```python
from build123d import *

# Parameters (mm, degrees)
CROQUIS1_R                                           = 8.5
SALIENTE_EXTRUIR1_DEPTH                              = 6
SALIENTE_EXTRUIR2_DEPTH                              = 5
REFRENTADO_PARA_TORNILLO_CON_CABEZA_TRON_D           = 4.5
REFRENTADO_PARA_TORNILLO_CON_CABEZA_TRON_CBORE_D     = 6
REFRENTADO_PARA_TORNILLO_CON_CABEZA_TRON_CBORE_DEPTH = 3.1
CHAFL_N1_SIZE                                        = 5
REDONDEO1_R                                          = 10
CHAFL_N2_SIZE                                        = 2
REDONDEO2_R                                          = 5
REDONDEO3_R                                          = 5
REDONDEO4_R                                          = 5
REDONDEO5_R                                          = 5


with BuildPart() as part:
    # Croquis1 → Saliente-Extruir1 (new body)
    with BuildSketch(Plane.XY):
        Polygon((-22.5, 0), (22.5, 0), (22.5, 17), (13, 17), (13, 34), (-13, 34), (-13, 17), (-22.5, 17), align=None)
        with Locations((0, 22)):
            Circle(CROQUIS1_R, mode=Mode.SUBTRACT)
    extrude(amount=SALIENTE_EXTRUIR1_DEPTH)

    # Croquis2 → Saliente-Extruir2 (add)
    with BuildSketch(Plane.XY.offset(6)):
        Polygon((22.5, 0), (22.5, 17), (13, 17), (13, 34), (-13, 34), (-13, 17), (-22.5, 17), (-22.5, 0), align=None)
    extrude(amount=SALIENTE_EXTRUIR2_DEPTH)

    # Refrentado para tornillo con cabeza troncocónica de M41 (through all)
    with Locations(Plane(origin=(17, 17, 5.5), x_dir=(1, 0, 0), z_dir=(0, 1, 0))):
        with Locations((0, 0), (-34, 0)):
            CounterBoreHole(REFRENTADO_PARA_TORNILLO_CON_CABEZA_TRON_D / 2, REFRENTADO_PARA_TORNILLO_CON_CABEZA_TRON_CBORE_D / 2, REFRENTADO_PARA_TORNILLO_CON_CABEZA_TRON_CBORE_DEPTH)

    # Chaflán1
    # the kernel refuses this chamfer: 5 mm, written as the material it adds along each edge
    with BuildSketch(Plane(origin=(-13, 17, 11), x_dir=(-0.9996219169112968, -0.02749587661058561, 0), z_dir=(0, 0, -1))) as chafl_n1_piece_1_section:
        Polygon((CHAFL_N1_SIZE * 0.999621916911, CHAFL_N1_SIZE * 0.0274958766106), (-CHAFL_N1_SIZE * 0.0274958766106, CHAFL_N1_SIZE * 0.999621916911), (0, 0), align=None)
    chafl_n1_piece_1 = extrude(amount=11, mode=Mode.PRIVATE)
    chafl_n1_piece_1 = chafl_n1_piece_1 - Plane(origin=(-17, 17.70483049, 5.5), x_dir=(1, 0, 0), z_dir=(0, 1, 0)) * Cylinder(3, 42, mode=Mode.PRIVATE)
    add(chafl_n1_piece_1)
    with BuildSketch(Plane(origin=(13, 17, 0), x_dir=(0.9996219169112968, -0.027495876610585626, 0), z_dir=(0, 0, 1))) as chafl_n1_piece_2_section:
        Polygon((CHAFL_N1_SIZE * 0.999621916911, CHAFL_N1_SIZE * 0.0274958766106), (-CHAFL_N1_SIZE * 0.0274958766106, CHAFL_N1_SIZE * 0.999621916911), (0, 0), align=None)
    chafl_n1_piece_2 = extrude(amount=11, mode=Mode.PRIVATE)
    chafl_n1_piece_2 = chafl_n1_piece_2 - Plane(origin=(17, 17.70483049, 5.5), x_dir=(1, 0, 0), z_dir=(0, 1, 0)) * Cylinder(3, 42, mode=Mode.PRIVATE)
    add(chafl_n1_piece_2)

    # Redondeo1
    redondeo1_edges = [part.edges().sort_by_distance(p)[0] for p in [
        (-13, 34, 5.5),
        (13, 34, 5.5),
    ]]
    fillet(redondeo1_edges, radius=REDONDEO1_R)

    # Chaflán2
    chafl_n2_edges = [part.edges().sort_by_distance(p)[0] for p in [
        (-22.5, 17, 5.5),
        (22.5, 17, 5.5),
    ]]
    chamfer(chafl_n2_edges, length=CHAFL_N2_SIZE)

    # Redondeo2
    # the kernel refuses this fillet: 5 mm, written as the material it takes off along each edge
    with BuildSketch(Plane(origin=(22.5, -12.5, 11), x_dir=(0, 0, -1), z_dir=(0, 1, 0))) as redondeo2_piece_1:
        with BuildLine():
            CenterArc((REDONDEO2_R, REDONDEO2_R), REDONDEO2_R, 180, 90)
            Line((0, REDONDEO2_R), (0, 0))
            Line((0, 0), (REDONDEO2_R, 0))
        make_face()
    extrude(amount=40, mode=Mode.SUBTRACT)

    # Redondeo3
    redondeo3_edges = [part.edges().sort_by_distance(p)[0] for p in [
        (-22.5, 7.5, 0),
    ]]
    fillet(redondeo3_edges, radius=REDONDEO3_R)

    # Redondeo4
    # the kernel refuses this fillet: 5 mm, written as the material it takes off along each edge
    with BuildSketch(Plane(origin=(22.5, -12.5, 0), x_dir=(-1, 0, 0), z_dir=(0, 1, 0))) as redondeo4_piece_1:
        with BuildLine():
            CenterArc((REDONDEO4_R, REDONDEO4_R), REDONDEO4_R, 180, 90)
            Line((0, REDONDEO4_R), (0, 0))
            Line((0, 0), (REDONDEO4_R, 0))
        make_face()
    extrude(amount=40, mode=Mode.SUBTRACT)

    # Redondeo5
    # the kernel refuses this fillet: 5 mm, written as the material it takes off along each edge
    with BuildSketch(Plane(origin=(-22.5, 27.5, 11), x_dir=(0, 0, -1), z_dir=(0, -1, 0))) as redondeo5_piece_1:
        with BuildLine():
            CenterArc((REDONDEO5_R, REDONDEO5_R), REDONDEO5_R, 180, 90)
            Line((0, REDONDEO5_R), (0, 0))
            Line((0, 0), (REDONDEO5_R, 0))
        make_face()
    extrude(amount=40, mode=Mode.SUBTRACT)


solid = part.part
```
Could you check a few things on this model? Use its own coordinates, in mm. A direction names the side the tool comes from. Round coordinates to 2 decimals unless told otherwise and drop trailing zeros. Loops run counter-clockwise (first coordinate to the right, second up) from the corner with the lowest first, then second, coordinate; pieces in that order, holes last. Notation, with made-up numbers: (49, -38.5) -> (59, -38.5) arc R23 ccw to (59, -24.5) -> close; hole circle Ø8 at (3.25, 71.25). An arc over 180 degrees is marked (long way). Put each result on its own line as item: value.
Q1. Please list where these lines run through material, in increasing order: line 1 (Z direction, x = -17, y = 5.5); line 2 (Z direction, x = 17, y = 17.75); line 3 (X direction, y = 4, z = 5). Write a range as from..to.
Checks:
line 1: 0..3.25, 7.75..11
line 2: 0..2.5, 8.5..11
line 3: -22.5..-19.19, -14.81..14.81, 19.19..22.5
Q2. I want a section at C-C on y = 6.5. Write out the boundary of the cut face in (x, z).
Checks:
outline: (-22.5, 5) arc R5 ccw to (-17.5, 0) -> (17.5, 0) arc R5 ccw to (22.5, 5) -> (22.5, 6) arc R5 ccw to (17.5, 11) -> (-17.5, 11) arc R5 ccw to (-22.5, 6) -> close; hole circle Ø4.5 at (-17, 5.5); hole circle Ø4.5 at (17, 5.5)
Q3. For pin 1 Ø5 at (x, y) = (15, 24.5) entering from +Z; pin 2 Ø3 at (x, z) = (-19.5, 4.5) entering from +Y; pin 3 Ø1.6 at (y, z) = (23.5, 4.5) entering from -X; pin 4 Ø3 at (x, z) = (16.5, 8.5) entering from +Y, each with a flat end and sliding along its axis, tell me the tip position at first contact or that it passes through.
Checks:
pin 1: z = 11
pin 2: y = 17
pin 3: x = -13
pin 4: y = 20
Q4. Which directions (+Z, -Z, +X, -X, +Y, -Y) give clear straight access to the entire face, cutting with the end or side of a thin tool? Please do faces 5 (the cylindrical face through (14, 16.8, 5.4)), 6 (the cylindrical face through (-21, 8.87, 9.57)).
Checks:
face 5: +Y
face 6: +Z, -X, +Y, -Y
Q5. I want a section at A-A on z = 5.5. Give the number of separate pieces and of enclosed holes in the cut face, and give its area (3 significant figures).
Checks:
separate pieces: 3
enclosed holes: 1
area: 780 mm2
Q6. I want a section at D-D on x = 0. Write out the boundary of the cut face in (y, z), and give its area (3 significant figures).
Checks:
outline: (0, 0) -> (13.5, 0) -> (13.5, 6) -> (30.5, 6) -> (30.5, 0) -> (34, 0) -> (34, 11) -> (0, 11) -> close
area: 272 mm2
Q7. I want a section at B-B on x = 17. Write out the boundary of the cut face in (y, z), and give its area (3 significant figures).
Checks:
outline: (0, 0) -> (18, 0) -> (18, 2.5) -> (13.9, 2.5) -> (13.9, 3.25) -> (0, 3.25) -> close; (0, 7.75) -> (13.9, 7.75) -> (13.9, 8.5) -> (18, 8.5) -> (18, 11) -> (0, 11) -> close
area: 111 mm2
Q8. Thinking about a two-plate mould opening in Y: for faces 1 (the flat face through (-13, 23, 5)), 2 (the flat face through (20, 17, 7)), 3 (the cylindrical face through (-1.84, 13.7, 2.96)), 4 (the flat face through (0, 22, 6)), which applies, pulls with the +Y half, pulls with the -Y half, needs draft (parallel to the pull), parting line crosses it, or undercut?
Checks:
face 1: needs draft
face 2: pulls with the +Y half
face 3: undercut
face 4: undercut
